For this review, take the finished solid that the model builds, in its own axes (mm). A direction names the side the tool comes from. Give positions to 0.01 mm unless a question says otherwise; leave off trailing zeros. Write each loop counter-clockwise with the first axis right and the second up, starting at its lowest first coordinate (ties: lowest second). Pieces come first, ordered by that corner, then holes. Notation, with made-up numbers: (61.5, 2.5) -> (72.5, 2.5) arc R35 ccw to (72.5, 34.5) -> close; hole circle Ø4 at (-13.75, 55). An arc over 180 degrees is marked (long way). Return JSON: item names as keys, results as strings.
from build123d import *

# Parameters (mm, degrees)
F0_R      = 26
F0_R_2    = 6.25
F1_DEPTH  = 30
F3_DEPTH  = 25
F4_DEPTH  = 22
F5_R      = 1.5
F6_DEPTH  = 25
F7_R      = 1.5
F8_DEPTH  = 25
F9_R      = 6.5
F10_DEPTH = 10


with BuildPart() as f1:
    # F0 (on Top) → F1 (new body)
    with BuildSketch(Plane.XY):
        Circle(F0_R)
        Circle(F0_R_2, mode=Mode.SUBTRACT)
        Circle(F0_R_2)
    extrude(amount=F1_DEPTH)

    # F0 (on Top) → F3 (cut)
    with BuildSketch(Plane.XY):
        Circle(F0_R_2)
    extrude(amount=F3_DEPTH, mode=Mode.SUBTRACT)

    # F2 (on face) → F4 (cut)
    with BuildSketch(Plane.XY.offset(30)):
        with BuildLine():
            Line((6.75, -2.2810359489), (6.75, 2.2810359489))
            ThreePointArc((6.75, 2.2810359489), (5.038135816, 5.038135816), (2.2810359489, 6.75))
            Line((2.2810359489, 6.75), (-2.2810359489, 6.75))
            ThreePointArc((-2.2810359489, 6.75), (-5.038135816, 5.038135816), (-6.75, 2.2810359489))
            Line((-6.75, 2.2810359489), (-6.75, -2.2810359489))
            ThreePointArc((-6.75, -2.2810359489), (-5.038135816, -5.038135816), (-2.2810359489, -6.75))
            Line((-2.2810359489, -6.75), (2.2810359489, -6.75))
            ThreePointArc((2.2810359489, -6.75), (5.038135816, -5.038135816), (6.75, -2.2810359489))
        make_face()
        with BuildLine():
            Line((-6.75, -2.2810359489), (-6.75, 2.2810359489))
            ThreePointArc((-6.75, 2.2810359489), (-7.125, 0), (-6.75, -2.2810359489))
        make_face()
        with BuildLine():
            ThreePointArc((-2.2810359489, -6.75), (0, -7.125), (2.2810359489, -6.75))
            Line((2.2810359489, -6.75), (-2.2810359489, -6.75))
        make_face()
    extrude(amount=-F4_DEPTH, mode=Mode.SUBTRACT)

    # F5 (on face) → F6 (cut)
    with BuildSketch(Plane(origin=(6.75, 0, 0), x_dir=(0, -1, 0), z_dir=(-1, 0, 0))):
        with Locations((0, 19)):
            Circle(F5_R)
    extrude(amount=-F6_DEPTH, mode=Mode.SUBTRACT)

    # F7 (on face) → F8 (cut)
    with BuildSketch(Plane.XZ.offset(-6.75)):
        with Locations((0, 19)):
            Circle(F7_R)
    extrude(amount=-F8_DEPTH, mode=Mode.SUBTRACT)

    # F9 (on face) → F10 (cut)
    with BuildSketch(Plane.XY):
        with Locations((-7.8439684669, 16.2009925218)):
            Circle(F9_R)
        with Locations((10.1084868569, 14.8935722197)):
            Circle(F9_R)
        with Locations((17.9524553238, -1.3074203021)):
            Circle(F9_R)
        with Locations((7.8439684669, -16.2009925218)):
            Circle(F9_R)
        with Locations((-10.1084868569, -14.8935722197)):
            Circle(F9_R)
        with Locations((-17.9524553238, 1.3074203021)):
            Circle(F9_R)
    extrude(amount=F10_DEPTH, mode=Mode.SUBTRACT)


solid = f1.part
1. For faces 4 (the flat face through (-10, -15, 10)), 5 (the flat face through (2, 6.75, 19)), 6 (the cylindrical face through (-0.195, 16.241, 20.487)), list the 3-axis set-ups (+Z, -Z, +X, -X, +Y, -Y) from which the entire face can be reached by the end or side of a thin tool; tool diameter is ignored.
Results found:
{"face 4": "-Z", "face 5": "+Z", "face 6": "+Y"}
2. Add section B-B, the plane x = 0. State the section outline as (y, z) points (3 decimals), plus the area to 3 significant figures.
Results found:
{"outline": "(-26, 0) -> (-6.25, 0) -> (-6.25, 8) -> (-7.125, 8) -> (-7.125, 30) -> (-26, 30) -> close; (6.25, 0) -> (26, 0) -> (26, 17.5) -> (6.75, 17.5) -> (6.75, 8) -> (6.25, 8) -> close; (6.75, 20.5) -> (26, 20.5) -> (26, 30) -> (6.75, 30) -> close", "area": "1,100 mm²"}
3. To check wall thickness, follow probe 1 along Y at (x, z) = (-7, 5); probe 2 along Z at (x, y) = (-9.5, -9.5); probe 3 along X at (y, z) = (-11.5, 1). State the ranges of each line that lie inside material, in increasing order.
Results found:
{"probe 1": "y = -25.04 to -20.6, -9.19 to 9.76, 22.65 to 25.04", "probe 2": "z = 10 to 30", "probe 3": "x = -23.32 to -15.65, -4.56 to 3.36, 12.33 to 23.32"}
4. For pin 1 (5 mm diameter, centred on x = -12.5, z = 18.5, fed in from +Y); pin 2 (1.8 mm diameter, centred on y = 0, z = 19, fed in from +X); pin 3 (4 mm diameter, centred on y = -7.5, z = 14, fed in from -X), all flat-tipped, find the tip position at first contact; note any pin that passes through.
Results found:
{"pin 1": "stops at y = 24", "pin 2": "stops at x = -7.07", "pin 3": "stops at x = -25.41"}
5. Add section D-D, the plane z = 19. State the section outline as (x, y) points (3 decimals).
Results found:
{"outline": "(-2.281, 6.75) -> (-1.5, 6.75) -> (-1.5, 25.957) arc R26 ccw (long way) to (25.957, -1.5) -> (6.75, -1.5) -> (6.75, -2.281) arc R7.125 cw (long way) to start; (1.5, 6.75) -> (2.281, 6.75) arc R7.125 cw to (6.75, 2.281) -> (6.75, 1.5) -> (25.957, 1.5) arc R26 ccw to (1.5, 25.957) -> close"}
6. Add section C-C, the plane y = 0. State the section outline as (x, z) points (3 decimals), plus the area to 3 significant figures.
Results found:
{"outline": "(-26, 0) -> (-24.32, 0) -> (-24.32, 10) -> (-11.585, 10) -> (-11.585, 0) -> (-6.25, 0) -> (-6.25, 8) -> (-7.125, 8) -> (-7.125, 30) -> (-26, 30) -> close; (6.25, 0) -> (11.585, 0) -> (11.585, 10) -> (24.32, 10) -> (24.32, 0) -> (26, 0) -> (26, 17.5) -> (6.75, 17.5) -> (6.75, 8) -> (6.25, 8) -> close; (6.75, 20.5) -> (26, 20.5) -> (26, 30) -> (6.75, 30) -> close", "area": "842 mm²"}
7. Add section A-A, the plane z = 15.5. State the section outline as (x, y) points (3 decimals).
Results found:
{"outline": "circle Ø52 at (0, 0); hole (-2.281, 6.75) arc R7.125 ccw (long way) to (6.75, -2.281) -> (6.75, 2.281) arc R7.125 ccw to (2.281, 6.75) -> close"}
8. The part is to be moulded in two halves that separate along X. For faces 1 (the flat face through (5.4, -5.4, 30)), 2 (the flat face through (18, -1, 10)), 3 (the cylindrical face through (-20.633, -15.821, 14.79)), say which applies: +X half, -X half, draft (parallel to the pull), parting line (faces both ways), or undercut.
Results found:
{"face 1": "draft", "face 2": "undercut", "face 3": "parting line"}
